Read the model definition and answer for the solid it produces. Units are mm, in the model's axes. A direction names the side the tool comes from. Coordinates: 2 decimals unless noted, no trailing zeros. Write each loop counter-clockwise with the first axis right and the second up, starting at its lowest first coordinate (ties: lowest second). Pieces come first, ordered by that corner, then holes. Notation, with made-up numbers: (86.5, -18) -> (128.5, -18) arc R36 ccw to (128.5, 19) -> close; hole circle Ø5 at (47.5, -11). An arc over 180 degrees is marked (long way). Use CSV: the item, a comma, the result in double quotes. Start each with the question number.
from build123d import *

# Parameters (mm, degrees)
SKETCH1_R                   = 9.525
BOSS_EXTRUDE1_DEPTH         = 101.6
BOSS_EXTRUDE2_DEPTH         = 13.096875
F_1_2_13_TAPPED_HOLE1_D     = 10.71626
F_1_2_13_TAPPED_HOLE1_DEPTH = 25.4
F_1_2_13_TAPPED_HOLE1_TIP   = 3.219489309


with BuildPart() as part:
    # Sketch1 → Boss-Extrude1 (new body)
    with BuildSketch(Plane(origin=(0, 0, 0), x_dir=(1, 0, 0), z_dir=(0, 1, 0))):
        with Locations(Location((0, 0, 0), (0, 0, 270))):
            Circle(SKETCH1_R)
    extrude(amount=BOSS_EXTRUDE1_DEPTH)

    # Sketch4 → Boss-Extrude2 (add)
    with BuildSketch(Plane(origin=(0, 101.6, 0), x_dir=(1, 0, 0), z_dir=(0, 1, 0))):
        Polygon((0, 10.998522628), (9.525, 5.499261314), (9.525, -5.499261314), (0, -10.998522628), (-9.525, -5.499261314), (-9.525, 5.499261314), align=None)
    extrude(amount=BOSS_EXTRUDE2_DEPTH)

    # Sketch5 → Revolve2 (revolve)
    with BuildSketch(Plane.XY, mode=Mode.PRIVATE) as revolve2_sk:
        with BuildLine():
            Line((0, 101.6), (-15.108296375, 101.6))
            ThreePointArc((-15.108296375, 101.6), (-15.875, 102.188312383), (-15.505171375, 103.081157664))
            Line((-15.505171375, 103.081157664), (0, 112.033072532))
            Line((0, 112.033072532), (0, 101.6))
        make_face()
    revolve(revolve2_sk.sketch.rotate(Axis((0, 101.6, 0), (0, 1, 0)), 180), axis=Axis((0, 101.6, 0), (0, 1, 0)))

    # 1/2-13 Tapped Hole1
    with Locations(Plane(origin=(0, 0, 0), x_dir=(-1, 0, 0), z_dir=(0, -1, 0))):
        with Locations((0, 0)):
            Hole(F_1_2_13_TAPPED_HOLE1_D / 2, depth=F_1_2_13_TAPPED_HOLE1_DEPTH)
            with Locations((0, 0, -(F_1_2_13_TAPPED_HOLE1_DEPTH + F_1_2_13_TAPPED_HOLE1_TIP / 2))):  # 118° drill point
                Cone(0, F_1_2_13_TAPPED_HOLE1_D / 2, F_1_2_13_TAPPED_HOLE1_TIP, mode=Mode.SUBTRACT)


solid = part.part
1) Find the intervals of material crossed by line 1 along Z through (x, y) = (2.5, 25); line 2 along Z through (x, y) = (3, 16); line 3 along Y through (x, z) = (7, 6.5), in increasing order.
2) Each of these flat-tipped pins is pushed along its axis until it touches: pin 1 (6 mm diameter, centred on y = 47, z = -11, fed in from -X); pin 2 (4 mm diameter, centred on x = -2, z = 10, fed in from +Y); pin 3 (9.5 mm diameter, centred on x = 0, z = 0, fed in from -Y); pin 4 (4.5 mm diameter, centred on y = 110.5, z = 0, fed in from +X) (3 decimals). Where does it stop, or does it pass through?
3) Section B-B, the plane y = 61.5 is taken. Give the vertices of the cut face in (x, z) (3 decimals), plus the area to 3 significant figures.
4) The mould has two halves that part along Z. Classify faces 1 (the face through (0.2, 28.06, 0.91)), 2 (the face through (-5.796, 50.089, -7.559)), 3 (the face through (2.472, 12.878, 4.754)), 4 (the face through (0, 114.697, 0)): pulls with the +Z half, pulls with the -Z half, needs draft (parallel to the pull), parting line crosses it, or undercut.
5) Section A-A, the plane y = 7.5 is taken. Give the vertices of the cut face in (x, z) (3 decimals), plus the area to 3 significant figures.
6) Which of the six approach directions +Z, -Z, +X, -X, +Y, -Y give full straight-line access (tool end or side, diameter ignored) to faces 5 (the face through (-4.696, 110.127, 8.287)), 6 (the face through (4.83, 110.13, 8.21)), 7 (the face through (0, 101.6, 10)), 8 (the face through (-4.83, 110.13, -8.21))?
The answers:
1,line 1,"z = -9.19 to -4.74, 4.74 to 9.19"
1,line 2,"z = -9.04 to -4.44, 4.44 to 9.04"
1,line 3,"y = 101.6 to 114.7"
2,pin 1,"stops at x = -5.17"
2,pin 2,"stops at y = 114.7"
2,pin 3,"stops at y = 25.77"
2,pin 4,"stops at x = 9.525"
3,outline,"circle Ø19.05 at (0, 0)"
3,area,"285 mm^2"
4,face 1,"undercut"
4,face 2,"parting line crosses it"
4,face 3,"undercut"
4,face 4,"needs draft"
5,outline,"circle Ø19.05 at (0, 0); hole circle Ø10.716 at (0, 0)"
5,area,"195 mm^2"
6,face 5,"+Z, -X, +Y"
6,face 6,"+Z, +X, +Y"
6,face 7,"-Y"
6,face 8,"-Z, -X, +Y"
